For this review, take the finished solid that the model builds, in its own axes (mm). Coordinates: 2 decimals unless noted, no trailing zeros. Write each loop counter-clockwise with the first axis right and the second up, starting at its lowest first coordinate (ties: lowest second). Pieces come first, ordered by that corner, then holes. Notation, with made-up numbers: (-22.75, 19.25) -> (-1.75, 19.25) arc R20 ccw to (-1.75, 41.25) -> close; hole circle Ø5 at (66, -4.75). An arc over 180 degrees is marked (long way). One line per item, written item: value. Start each with the question number.
1) For probe 1 along X at (y, z) = (0.8, -0.5); probe 2 along X at (y, z) = (0.75, 0.4); probe 3 along Z at (x, y) = (8.75, -0.9), list the stretches that pass through material, from the lowest coordinate up. Write a range as from..to.
2) Add section C-C (x = 8.25). State the section outline as (y, z) points, and give its area (3 significant figures).
3) Mouldability with a two-part tool opening along X and no side actions: class faces 1 (the cylindrical face through (1.6, 0.72, -0.23)), 2 (the flat face through (0, 1, 0)), 3 (the cylindrical face through (11, 0, 1)) as released by +X, released by -X, zero draft, split by the parting line, or undercut.
4) For pin 1 Ø1 at (x, y) = (4, 0.5) entering from +Z; pin 2 Ø2 at (x, z) = (14.5, -0.5) entering from +Y; pin 3 Ø2 at (x, z) = (7.5, -0.5) entering from -Y, all flat-tipped, find the tip position at first contact; note any pin that passes through.
5) Add section B-B (y = 0). State the section outline as (x, z) points, and give its area (3 significant figures).
6) Add section A-A (z = 0). State the section outline as (x, y) points.
Autodesk Inventor part; units mm, degrees
ref_plane "Work Plane1" through (33.575, 0, 0) normal (0, 0, -1) x (1, 0, 0)
ref_plane "YZ Plane" through (0, 0, 0) normal (1, 0, 0) x (0, 1, 0)
ref_plane "XZ Plane" through (0, 0, 0) normal (0, 1, 0) x (-1, 0, 0)
sketch "Sketch1" plane through (0, 0, 0) normal (0, 0, 1) x (1, 0, 0)
  line L0 (0, 0) -> (20, 0)
  line L1 (20, 0) -> (20, 1)
  line L2 (20, 1) -> (2, 1)
  line L3 (2, 1) -> (1.7546, 0.7546)
  line L4 (1.7546, 0.7546) -> (1.4454, 0.7546)
  line L5 (1.4454, 0.7546) -> (0.45, 1.75)
  line L6 (0.45, 1.75) -> (0, 1.75)
  line L7 (0, 1.75) -> (0, 0)
  line L8 (2, 1) -> (1.2, 1) construction
  line L9 (-4, 0) -> (24, 0)
  line L10 (0, 2.1) -> (0, -0.35)
  dimension "d0" = 20
  dimension "d1" = 45
  dimension "d2" = 0.2454
  dimension "d3" = 18
  dimension "d4" = 1.2
  dimension "d5" = 1.5092
  dimension "d6" = 2
  dimension "d7" = 3.5
revolve "Body" add sketch "Sketch1" angle 360 about axis through (0, 0, 0) along (1, 0, 0)
sketch "Sketch2" plane through (0, 0, 0) normal (-1, 0, 0) x (0, 0, 1)
  line L0 (1.75, -0.35) -> (-1.75, -0.35)
  line L1 (-1.75, -0.35) -> (-1.75, 0.35)
  line L2 (-1.75, 0.35) -> (1.75, 0.35)
  line L3 (1.75, 0.35) -> (1.75, -0.35)
  line L4 (0, 0.35) -> (0, -0.35) construction
  line L5 (-1.75, 0) -> (1.75, 0) construction
  line L6 (0, 1.75) -> (0, 0)
  dimension "d15" = 0.7
  dimension "d16" = 3.5
extrude "Slot" cut sketch "Sketch2" against normal blind 0.4
thread "Thread"
chamfer "Chamfer1" distance 0.2454 distance2 0.1227 1 edges at (20, -1, 0) measured on face at (20, -0.379, 0.3759)
ref_plane "Work Plane1" through (33.575, 0, 0) normal (0, 0, -1) x (1, 0, 0)
equation "\"d0\" = NLG"
equation "\"d1\" = 0.5 * SEWI"
equation "\"d2\" = GAL"
equation "\"d3\" = GEL"
equation "\"d4\" = KOH"
equation "\"d5\" = BDM"
equation "\"d6\" = GD"
equation "\"d7\" = KOD"
equation "\"d15\" = SBR"
equation "\"d16\" = KOD"
equation "\"d8\" = STI"
equation "\"d10\" = GEL"
equation "\"d12\" = -0.5 * SPD + 0.5 * GD"
equation "\"d13\" = 0.5 * GAL"
equation "\"NLG\" = 20"
equation "\"GAL\" = 0.61345 * PTC"
equation "\"GEL\" = 18"
equation "\"KOH\" = 1.2"
equation "\"KOD\" = 3.5"
equation "\"SEWI\" = 90deg"
equation "\"BDM\" = NND - 1.2269 * PTC"
equation "\"GD\" = NND"
equation "\"SBR\" = 0.7"
equation "\"STI\" = 0.4"
equation "\"SPD\" = NND - 1.2269 * PTC"
equation "\"GUL\" = 0.61345 * PTC"
equation "\"PTC\" = 0.4"
equation "\"EPV\" = 2.2"
equation "\"THREADDIA\" = 2"
equation "\"TOA\" = 30deg"
equation "\"RR\" = 0.2"
equation "\"NND\" = 2"
equation "\"GD1\" = THREADDIA - 1.2269 * PTC"
properties part number "AS 1427 - M2 x 20" material "Steel, Mild"
Numbers:
1. probe 1: 0..1.26, 1.94..19.91
1. probe 2: 0..1.35, 1.85..19.95
1. probe 3: -0.44..0.44
2. outline: circle Ø2 at (0, 0)
2. area: 3.14 mm²
3. face 1: undercut
3. face 2: released by -X
3. face 3: zero draft
4. pin 1: z = 1
4. pin 2: y = 1
4. pin 3: y = -1
5. outline: (0.4, -1.75) -> (0.45, -1.75) -> (1.45, -0.75) -> (1.75, -0.75) -> (2, -1) -> (19.88, -1) -> (20, -0.75) -> (20, 0.75) -> (19.88, 1) -> (2, 1) -> (1.75, 0.75) -> (1.45, 0.75) -> (0.45, 1.75) -> (0.4, 1.75) -> close
5. area: 39.5 mm²
6. outline: (0, -1.75) -> (0.45, -1.75) -> (1.45, -0.75) -> (1.75, -0.75) -> (2, -1) -> (19.88, -1) -> (20, -0.75) -> (20, 0.75) -> (19.88, 1) -> (2, 1) -> (1.75, 0.75) -> (1.45, 0.75) -> (0.45, 1.75) -> (0, 1.75) -> (0, 0.35) -> (0.4, 0.35) -> (0.4, -0.35) -> (0, -0.35) -> close
